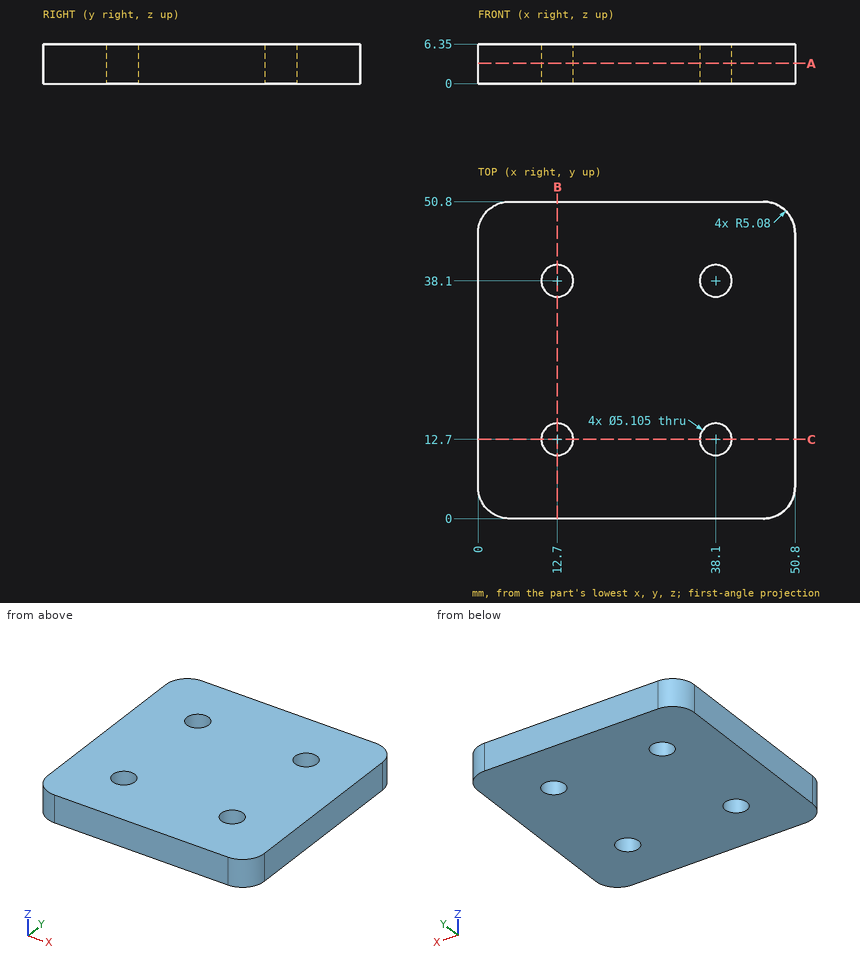
Input: dimensioned drawing with shaded views. Units: mm. Origin: part minimum x, y, z. Round coordinates to 2 decimals unless told otherwise and drop trailing zeros. Loops run counter-clockwise (first coordinate to the right, second up) from the corner with the lowest first, then second, coordinate; pieces in that order, holes last. Notation, with made-up numbers: (51, 76.25) -> (67, 76.25) arc R11 cw to (67, 91.25) -> close; hole circle Ø3 at (28, -19.75). An arc over 180 degrees is marked (long way). Answer as a JSON object with one key per item and string values. Group by question number.
Q1. Ray query, line 1 (Y direction, x = 12.7, z = 2.75); line 2 (Y direction, x = 13.5, z = 4.5) (1 decimal); line 3 (X direction, y = 36, z = 0.75). Return the intervals inside material, ascending. Write a range as from..to.
Q2. Section query B-B (x = 12.7). Output: boundary loops of the cut face in (y, z).
Q3. Section query A-A (z = 3.25). Output: boundary loops of the cut face in (x, y) (1 decimal).
Completed:
{
 "1": {"line 1": "0..10.15, 15.25..35.55, 40.65..50.8", "line 2": "0..10.3, 15.1..35.7, 40.5..50.8", "line 3": "0..11.25, 14.15..36.65, 39.55..50.8"},
 "2": {"outline": "(0, 0) -> (10.15, 0) -> (10.15, 6.35) -> (0, 6.35) -> close; (15.25, 0) -> (35.55, 0) -> (35.55, 6.35) -> (15.25, 6.35) -> close; (40.65, 0) -> (50.8, 0) -> (50.8, 6.35) -> (40.65, 6.35) -> close"},
 "3": {"outline": "(0, 5.1) arc R5.1 ccw to (5.1, 0) -> (45.7, 0) arc R5.1 ccw to (50.8, 5.1) -> (50.8, 45.7) arc R5.1 ccw to (45.7, 50.8) -> (5.1, 50.8) arc R5.1 ccw to (0, 45.7) -> close; hole circle Ø5.1 at (12.7, 12.7); hole circle Ø5.1 at (12.7, 38.1); hole circle Ø5.1 at (38.1, 12.7); hole circle Ø5.1 at (38.1, 38.1)"}
}
